Geometry: see drawing. Coordinates: mm, zero at the bounding-box minimum. A direction names the side the tool comes from. Give positions to 0.01 mm unless a question says otherwise; leave off trailing zeros. Loops run counter-clockwise (first coordinate to the right, second up) from the corner with the lowest first, then second, coordinate; pieces in that order, holes last. Notation, with made-up numbers: M -2,-37.5 L 9,-37.5 A24 ccw 9,-0.5 Z; hole C 13.5,24.25 d11. An arc over 180 degrees is marked long. Put each result on its own line as item: value.
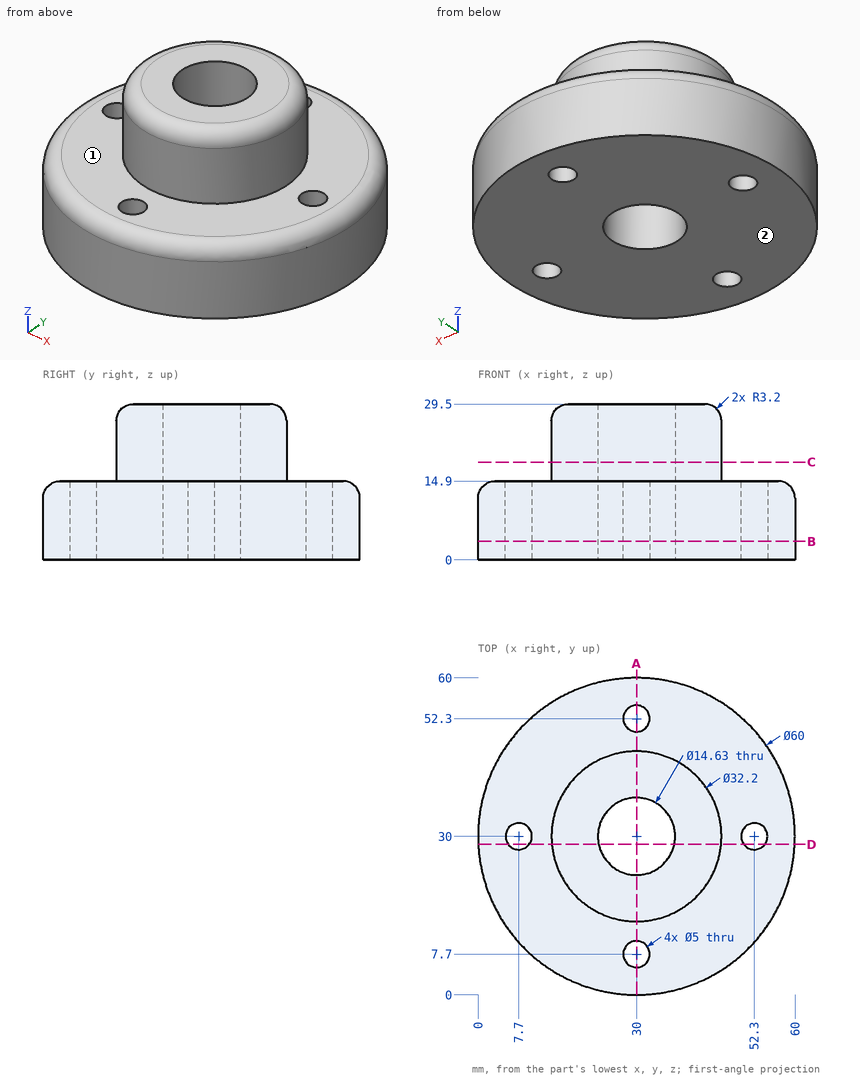
Item 1: Set-up query: the marked faces 1 and 2. Return all of +Z, -Z, +X, -X, +Y, -Y with unobstructed straight access to the full face (end or side cutting, diameter ignored); none if empty.
Output values:
face 1: +Z
face 2: -Z, +X, -X, +Y, -Y
Item 2: Section A-A on x = 30. Output: boundary loops of the cut face in (y, z) (3 decimals).
Output values:
outline: M 0,0 L 5.2,0 L 5.2,14.9 L 3.2,14.9 A3.2 ccw 0,11.7 Z; M 10.2,0 L 22.685,0 L 22.685,29.5 L 17.1,29.5 A3.2 ccw 13.9,26.3 L 13.9,14.9 L 10.2,14.9 Z; M 37.315,0 L 49.8,0 L 49.8,14.9 L 46.1,14.9 L 46.1,26.3 A3.2 ccw 42.9,29.5 L 37.315,29.5 Z; M 54.8,0 L 60,0 L 60,11.7 A3.2 ccw 56.8,14.9 L 54.8,14.9 Z
Item 3: Section D-D on y = 28.5. Count the separate pieces of the cut face and the enclosed holes in it, then the cut area to 3 significant figures.
Output values:
separate pieces: 4
enclosed holes: 0
area: 811 mm²
Item 4: Section B-B on z = 3.5. Output: boundary loops of the cut face in (x, y) (3 decimals), then the cut area to 3 significant figures.
Output values:
outline: C 30,30 d60; hole C 7.7,30 d5; hole C 30,30 d14.63; hole C 30,7.7 d5; hole C 30,52.3 d5; hole C 52.3,30 d5
area: 2,580 mm²
Item 5: Line query: probe 1 along Y at (x, z) = (30, 6) (3 decimals); probe 2 along Y at (x, z) = (30, 18) (3 decimals); probe 3 along Z at (x, y) = (11, 37). Output: solid intervals per line, ascending. Write a range as [from, to].
Output values:
probe 1: [0, 5.2], [10.2, 22.685], [37.315, 49.8], [54.8, 60]
probe 2: [13.9, 22.685], [37.315, 46.1]
probe 3: [0, 14.9]
Item 6: Section C-C on z = 18.5. Output: boundary loops of the cut face in (x, y) (3 decimals).
Output values:
outline: C 30,30 d32.2; hole C 30,30 d14.63
Item 7: Pin query (flat end, axial travel): pin 1 Ø6 at (y, z) = (14, 6) entering from -X; pin 2 Ø10 at (y, z) = (23.5, 14.5) entering from -X; pin 3 Ø3 at (y, z) = (29.5, 15) entering from -X. Return the tip coordinate at first contact, or that it passes through.
Output values:
pin 1: x = 2.96
pin 2: x = 0.09
pin 3: x = 0.56
